from build123d import *

# Parameters (mm, degrees)
F1_DEPTH = 44.45
F2_R     = 12.7
F3_DEPTH = 45.72
F4_W     = 12.7
F4_H     = 63.5
F5_DEPTH = 127
F6_R     = 5.08
F7_DEPTH = 11.43


with BuildPart() as f1:
    # F0 (on Front) → F1 (new body)
    with BuildSketch(Plane.XZ):
        with BuildLine():
            Line((0, 12.7), (0, 0))
            Line((0, 0), (63.5, 0))
            Line((63.5, 0), (63.5, 12.7))
            Line((63.5, 12.7), (44.45, 12.7))
            Line((44.45, 12.7), (44.45, 21.59))
            Line((44.45, 21.59), (95.25, 21.59))
            Line((95.25, 21.59), (95.25, 34.29))
            Line((95.25, 34.29), (78.74, 34.29))
            Line((78.74, 34.29), (53.000424, 73.603284))
            ThreePointArc((53.000424, 73.603284), (31.75, 85.09), (10.499576, 73.603284))
            Line((10.499576, 73.603284), (-15.24, 34.29))
            Line((-15.24, 34.29), (-31.75, 34.29))
            Line((-31.75, 34.29), (-31.75, 21.59))
            Line((-31.75, 21.59), (19.05, 21.59))
            Line((19.05, 21.59), (19.05, 12.7))
            Line((19.05, 12.7), (0, 12.7))
        make_face()
    extrude(amount=F1_DEPTH)

    # F2 (on face) → F3 (cut)
    with BuildSketch(Plane.XZ.offset(44.45)):
        with Locations((31.75, 59.69)):
            Circle(F2_R)
    extrude(amount=-F3_DEPTH, mode=Mode.SUBTRACT)

    # F4 (on face) → F5 (join)
    with BuildSketch(Plane.YZ.offset(95.25)):
        with Locations((6.35, 53.34)):
            Rectangle(F4_W, F4_H)
    extrude(amount=-F5_DEPTH)

    # F6 (on face) → F7 (cut)
    with BuildSketch(Plane.XY.offset(85.09)):
        with Locations((31.75, -22.225)):
            Circle(F6_R)
    extrude(amount=-F7_DEPTH, mode=Mode.SUBTRACT)


solid = f1.part
Model file for the job. Use its own axes, mm. A direction names the side the tool comes from. Round coordinates to 2 decimals unless told otherwise and drop trailing zeros. Order: outer loops, then holes, each group sorted by start corner. A loop starts at its lowest first (then second) coordinate and runs counter-clockwise, first axis right, second up. Notation, with made-up numbers: M 83,-31.5 L 91,-31.5 A28 ccw 91,3.5 Z; hole C 29,50 d5. An arc over 180 degrees is marked long. Write each question's results on one line, items separated by ' | '. Start each with the question number.
(1) Saw through at D-D, the plane z = 55.5. Give the cut face in (x, y), then the cut area to 3 significant figures.
(2) Which spindle directions (+Z, -Z, +X, -X, +Y, -Y) get a long thin tool onto all of the face, cutting with end or side? Do faces 1 (the face through (10, -22, 12.7)), 2 (the face through (63.5, -22, 6)), 3 (the face through (-23, -22, 34.29)), 4 (the face through (66.05, -21.91, 53.67)), 5 (the face through (31.09, -17.19, 79.46)). Say none if no direction does.
(3) Saw through at A-A, the plane x = 2.5. Give the cut face in (y, z).
(4) Probe probe 1 along Z at (x, y) = (31.75, -15.5); probe 2 along Z at (x, y) = (31, -26); probe 3 along Y at (x, z) = (68, 82.5). List the from-to ranges inside material, lowest first. Write a range as from..to.
(5) Two-plate mould, pull along X, no slides. Class faces 6 (the face through (47, -16, 21.59)), 7 (the face through (32, 0, 60)), 8 (the face through (-31.75, 3, 40)): pulls with the +X half, pulls with the -X half, needs draft (parallel to the pull), parting line crosses it, or undercut.
(6) Saw through at C-C, the plane z = 15.5. Give the cut face in (x, y).
(7) Saw through at B-B, the plane z = 44. Give the cut face in (x, y).
(8) Drop flat-ended pins along their axis: pin 1 (5 mm diameter, centred on x = 83, y = -26, fed in from +Z); pin 2 (10 mm diameter, centred on x = 2.5, y = -20, fed in from +Z); pin 3 (7 mm diameter, centred on y = -18, z = 15, fed in from -X). Give the stop position or say it passes through.
Established:
1) outline: M -31.75,0 L -1.35,0 L -1.35,-44.45 L 19.76,-44.45 L 19.76,0 L 43.74,0 L 43.74,-44.45 L 64.85,-44.45 L 64.85,0 L 95.25,0 L 95.25,12.7 L -31.75,12.7 Z | area: 3,490 mm^2
2) face 1: -X, +Y, -Y | face 2: -Z, +X, +Y, -Y | face 3: +Z, -X, -Y | face 4: +Z, +X, -Y | face 5: +Z
3) outline: M -44.45,0 L 0,0 L 0,12.7 L -44.45,12.7 Z; M -44.45,21.59 L 12.7,21.59 L 12.7,85.09 L 0,85.09 L 0,61.39 L -44.45,61.39 Z
4) probe 1: z = 0..46.99, 72.39..85.09 | probe 2: z = 0..47.01, 72.37..73.66 | probe 3: y = 0..12.7
5) face 6: needs draft | face 7: undercut | face 8: pulls with the -X half
6) outline: M 19.05,-44.45 L 44.45,-44.45 L 44.45,0 L 19.05,0 Z
7) outline: M -31.75,0 L -8.88,0 L -8.88,-44.45 L 72.38,-44.45 L 72.38,0 L 95.25,0 L 95.25,12.7 L -31.75,12.7 Z
8) pin 1: stops at z = 34.29 | pin 2: stops at z = 69.02 | pin 3: stops at x = 0
